```python
from build123d import *

# Parameters (mm, degrees)
F0_W      = 1.5
F0_H      = 1.5
F0_W_2    = 0.5
F0_H_2    = 0.435
F0_W_3    = 4.546262
F0_H_3    = 4
F0_H_4    = 2.065
F4_DEPTH  = 22
F5_SIZE2  = 2
F5_SIZE   = 0.5358983849
F6_R      = 0.5
F8_D      = 5
F8_DEPTH  = 10
F8_TIP    = 1.5021515476
F10_D     = 4
F10_DEPTH = 6
F10_TIP   = 1.2017212381
F12_DEPTH = 25


# Not quite as in the source:
# - ends of sketch curves that miss each other by under 0.0002 mm in the source are joined


with BuildPart() as f1:
    # F0 (on Top) → F1 (revolve)
    with BuildSketch(Plane.XY):
        with Locations((41.523095, 3.230684)):
            Rectangle(F0_W, F0_H)
        Polygon((33.773095, 5.681561), (33.773095, 2.480684), (37.5528260833, 2.480684), (36.226833, 5.980684), (36.226833, 9.980684), (33.773095, 5.730684), align=None)
        Polygon((36.226833, 5.980684), (37.5528260833, 2.480684), (39.4471019167, 2.480684), (40.773095, 5.980684), align=None)
        with Locations((42.523095, 2.263184)):
            Rectangle(F0_W_2, F0_H_2)
        Polygon((40.773095, 5.980684), (39.4471019167, 2.480684), (40.773095, 2.480684), (40.773095, 3.980684), align=None)
        with Locations((41.523095, 2.263184)):
            Rectangle(F0_W, F0_H_2)
        Polygon((42.273095, 3.980684), (42.273095, 2.480684), (42.773095, 2.480684), (42.773095, 3.480684), align=None)
        with Locations((38.499964, 7.980684)):
            Rectangle(F0_W_3, F0_H_3)
        with BuildLine():
            Line((40.773095, 2.045684), (40.773095, 0.7342315134))
            add(Edge.make_bspline(
                [(42.226833, -0.0193156), (42.2268322283, 0.4093938973), (40.773095, 0.7342315134)],
                knots=[3.141593, 3.141593, 3.141593, 3.8525916266, 3.8525916266, 3.8525916266], degree=2, weights=[1, 0.9374728154, 1]))
            Line((42.226833, -0.0193156), (42.273095, -0.019316))
            Line((42.273095, -0.019316), (42.273095, 2.045684))
            Line((42.273095, 2.045684), (40.773095, 2.045684))
        make_face()
        with Locations((42.523095, 1.013184)):
            Rectangle(F0_W_2, F0_H_4)
        Polygon((39.4471019167, 2.480684), (39.2822999192, 2.045684), (40.773095, 2.045684), (40.773095, 2.480684), align=None)
        with BuildLine():
            Line((33.773095, 0.730684), (33.773095, -0.019316))
            Line((33.773095, -0.019316), (34.273095, -0.019316))
            Line((34.273095, -0.019316), (38.499964, -0.019316))
            Line((38.499964, -0.019316), (38.0839828646, 1.0786791495))
            add(Edge.make_bspline(
                [(38.0839828646, 1.0786791495), (35.8841941746, 1.2164838646), (33.773095, 1.0344109623)],
                knots=[4.3976955436, 4.3976955436, 4.3976955436, 5.1336990724, 5.1336990724, 5.1336990724], degree=2, weights=[1, 0.9330480766, 1]))
            Line((33.773095, 1.0344109623), (33.773095, 0.730684))
        make_face()
        with BuildLine():
            Line((33.773095, 2.045684), (33.773095, 1.0344109623))
            add(Edge.make_bspline(
                [(38.0839828646, 1.0786791495), (35.8841941746, 1.2164838646), (33.773095, 1.0344109623)],
                knots=[4.3976955436, 4.3976955436, 4.3976955436, 5.1336990724, 5.1336990724, 5.1336990724], degree=2, weights=[1, 0.9330480766, 1]))
            Line((38.0839828646, 1.0786791495), (37.7176280808, 2.045684))
            Line((37.7176280808, 2.045684), (33.773095, 2.045684))
        make_face()
        Polygon((33.773095, 2.480684), (33.773095, 2.045684), (37.7176280808, 2.045684), (37.5528260833, 2.480684), align=None)
        with BuildLine():
            Line((37.7176280808, 2.045684), (38.0839828646, 1.0786791495))
            add(Edge.make_bspline(
                [(38.8919051119, 1.0152247595), (38.499964, 1.0526202094), (38.0839828646, 1.0786791495)],
                knots=[4.2521316371, 4.2521316371, 4.2521316371, 4.3976955436, 4.3976955436, 4.3976955436], degree=2, weights=[1, 0.9973525626, 1]))
            Line((38.8919051119, 1.0152247595), (39.2822999192, 2.045684))
            Line((39.2822999192, 2.045684), (37.7176280808, 2.045684))
        make_face()
        with BuildLine():
            Line((38.0839828646, 1.0786791495), (38.499964, -0.019316))
            Line((38.499964, -0.019316), (38.8919051119, 1.0152247595))
            add(Edge.make_bspline(
                [(38.8919051119, 1.0152247595), (38.499964, 1.0526202094), (38.0839828646, 1.0786791495)],
                knots=[4.2521316371, 4.2521316371, 4.2521316371, 4.3976955436, 4.3976955436, 4.3976955436], degree=2, weights=[1, 0.9973525626, 1]))
        make_face()
        with BuildLine():
            Line((38.8919051119, 1.0152247595), (38.499964, -0.019316))
            Line((38.499964, -0.019316), (40.773095, -0.019316))
            Line((40.773095, -0.019316), (40.773095, 0.7342315134))
            add(Edge.make_bspline(
                [(40.773095, 0.7342315134), (39.9803120127, 0.9113788897), (38.8919051119, 1.0152247595)],
                knots=[3.8525916266, 3.8525916266, 3.8525916266, 4.2521316371, 4.2521316371, 4.2521316371], degree=2, weights=[1, 0.9801122448, 1]))
        make_face()
        Polygon((37.5528260833, 2.480684), (37.7176280808, 2.045684), (39.2822999192, 2.045684), (39.4471019167, 2.480684), align=None)
        with BuildLine():
            Line((39.2822999192, 2.045684), (38.8919051119, 1.0152247595))
            add(Edge.make_bspline(
                [(40.773095, 0.7342315134), (39.9803120127, 0.9113788897), (38.8919051119, 1.0152247595)],
                knots=[3.8525916266, 3.8525916266, 3.8525916266, 4.2521316371, 4.2521316371, 4.2521316371], degree=2, weights=[1, 0.9801122448, 1]))
            Line((40.773095, 0.7342315134), (40.773095, 2.045684))
            Line((40.773095, 2.045684), (39.2822999192, 2.045684))
        make_face()
        with BuildLine():
            Line((40.773095, 0.7342315134), (40.773095, -0.019316))
            Line((40.773095, -0.019316), (42.226833, -0.019316))
            add(Edge.make_bspline(
                [(42.226833, -0.019316), (42.2268322283, 0.4093938973), (40.773095, 0.7342315134)],
                knots=[3.141593, 3.141593, 3.141593, 3.8525916266, 3.8525916266, 3.8525916266], degree=2, weights=[1, 0.9374728154, 1]))
        make_face()
    revolve(axis=Axis((20.5738751867, -0.019316, 0), (1, 0, 0)))

    # F3 (on face) → F4 (join)
    with BuildSketch(Plane(origin=(33.773095, 0, 0), x_dir=(0, -1, 0), z_dir=(-1, 0, 0))):
        with BuildLine():
            ThreePointArc((0.7512693785, 5.7032222692), (-0.000602262, 5.749965501), (-0.7521320187, 5.698014387))
            ThreePointArc((-0.7521320187, 5.698014387), (-2.4254688054, 2.4414028529), (-5.6797608355, 0.7635595739))
            ThreePointArc((-5.6797608355, 0.7635595739), (-5.7306746348, 0.0103778617), (-5.6824799161, -0.7429827264))
            ThreePointArc((-5.6824799161, -0.7429827264), (-2.4218166649, -2.4249412056), (-0.7499999869, -5.6908159978))
            ThreePointArc((-0.7499999869, -5.6908159978), (0, -5.739939), (0.7500000036, -5.690816125))
            ThreePointArc((0.7500000036, -5.690816125), (2.4284043129, -2.4183433129), (5.7008769978, -0.7399389869))
            ThreePointArc((5.7008769978, -0.7399389869), (5.7377061387, -0.3657424933), (5.75, 0.010061))
            ThreePointArc((5.75, 0.010061), (5.7377061387, 0.3858644933), (5.700877125, 0.7600610036))
            ThreePointArc((5.700877125, 0.7600610036), (2.4311698073, 2.43570162), (0.7512693785, 5.7032222692))
        make_face()
    extrude(amount=F4_DEPTH)

    # F5
    f5_edges = [f1.edges().sort_by_distance(p)[0] for p in [
        (11.773095, 0.000602, 5.749966),
        (11.773095, -5.737706, 0.385864),
        (11.773095, 0, -5.739939),
        (11.773095, 5.730675, 0.010378),
    ]]
    f5_side = f1.faces().sort_by_distance((11.773095, -0.002803, 0.008597))[0]
    chamfer(f5_edges, length=F5_SIZE, length2=F5_SIZE2, reference=f5_side)

    # F6
    f6_edges = [f1.edges().sort_by_distance(p)[0] for p in [
        (11.773095, 0.001201, 5.214061),
        (11.773095, 5.194775, 0.010692),
        (11.773095, -5.195822, 0.446281),
    ]]
    fillet(f6_edges, radius=F6_R)

    # F8
    with Locations(Plane.YZ.offset(42.773095)):
        with Locations((0, 0)):
            Hole(F8_D / 2, depth=F8_DEPTH)
            with Locations((0, 0, -(F8_DEPTH + F8_TIP / 2))):  # 118° drill point
                Cone(0, F8_D / 2, F8_TIP, mode=Mode.SUBTRACT)

    # F10
    with Locations(Plane(origin=(11.773095, 0, 0), x_dir=(0, -1, 0), z_dir=(-1, 0, 0))):
        with Locations((0, 0)):
            Hole(F10_D / 2, depth=F10_DEPTH)
            with Locations((0, 0, -(F10_DEPTH + F10_TIP / 2))):  # 118° drill point
                Cone(0, F10_D / 2, F10_TIP, mode=Mode.SUBTRACT)

    # F11 (on face) → F12 (cut)
    with BuildSketch(Plane.YZ.offset(40.773095)):
        with BuildLine():
            ThreePointArc((8, -5.9741585928), (9.4726058286, -3.1469699713), (9.980684, 0))
            ThreePointArc((9.980684, 0), (9.4726058286, 3.1469699713), (8, 5.9741585928))
            Line((8, 5.9741585928), (8, -5.9741585928))
        make_face()
        with BuildLine():
            ThreePointArc((-8, 6), (-4.476454623, 8.9421112724), (-0.009658, 9.9999953362))
            ThreePointArc((-0.009658, 9.9999953362), (-10.019316, 0), (-0.009658, -9.9999953362))
            ThreePointArc((-0.009658, -9.9999953362), (-4.476454623, -8.9421112724), (-8, -6))
            Line((-8, -6), (-8, 6))
        make_face()
    extrude(amount=-F12_DEPTH, mode=Mode.SUBTRACT)


solid = f1.part
```
The listing builds one solid part. Answer for the finished solid, in the listing's coordinates (mm). A direction names the side the tool comes from. Round coordinates to 2 decimals unless told otherwise and drop trailing zeros. Loops run counter-clockwise (first coordinate to the right, second up) from the corner with the lowest first, then second, coordinate; pieces in that order, holes last. Notation, with made-up numbers: (39.25, -11.5) - (84.25, -11.5) arc R24 ccw to (84.25, 15.5) - close; hole circle Ø2 at (-38, -6.75). An arc over 180 degrees is marked (long way). Return JSON: item names as keys, results as strings. Group by question number.
1. The mould has two halves that part along Z. Classify faces 5 (the flat face through (33.773, -3, -3)), 6 (the conical face through (33.89, -5.97, 0.26)), 7 (the conical face through (31.53, -0.09, -0.42)), 8 (the cylindrical face through (37.7, 0.54, -2.44)): pulls with the +Z half, pulls with the -Z half, needs draft (parallel to the pull), parting line crosses it, or undercut.
2. Each of these flat-tipped pins is pushed along its axis until it touches: P1, Ø4, axis at x = 20, z = 7.5, coming from the -Y side; P2, Ø1.5, axis at y = 3, z = 3.5, coming from the -X side; P3, Ø4, axis at x = 20, y = -4.5, coming from the +Z side. Where does it stop, or does it pass through?
3. Which of the six approach directions +Z, -Z, +X, -X, +Y, -Y give full straight-line access (tool end or side, diameter ignored) to faces 1 (the cylindrical face through (22.927, 2.459, -2.388)), 2 (the cylindrical face through (22.93, 2.39, 2.48)), 3 (the cylindrical face through (22.93, -2.47, 2.4)), 4 (the cylindrical face through (23.91, 0.01, -5.74))?
4. The part is cut by section A-A on x = 22.5. Determine the outline of the cut face in (y, z).
5. Consider probe 1 along Y at (x, z) = (14.75, 0); probe 2 along Y at (x, z) = (38.25, 0); probe 3 along Z at (x, y) = (14.1, 0). Determine where each line is inside the solid, lowest interval first.
Resolved:
{
 "1": {"face 5": "needs draft", "face 6": "parting line crosses it", "face 7": "undercut", "face 8": "undercut"},
 "2": {"P1": "stops at y = -0.79", "P2": "stops at x = 33.77", "P3": "stops at z = 2.37"},
 "3": {"face 1": "-Z, -X, +Y", "face 2": "+Z, -X, +Y", "face 3": "+Z, -X, -Y", "face 4": "-Z, -X"},
 "4": {"outline": "(-5.75, 0.01) arc R5.75 ccw to (-5.7, -0.74) arc R6 cw to (-0.75, -5.69) arc R5.75 ccw to (0.75, -5.69) arc R6 cw to (5.68, -0.74) arc R5.75 ccw to (5.68, 0.76) arc R6 cw to (0.75, 5.7) arc R5.75 ccw to (-0.75, 5.7) arc R6 cw to (-5.7, 0.76) arc R5.75 ccw to start"},
 "5": {"probe 1": "y = -5.75 to -2, 2 to 5.73", "probe 2": "y = -8 to -2.5, 2.5 to 8", "probe 3": "z = -5.74 to -2, 2 to 5.75"}
}
